```python
from build123d import *

# Parameters (mm, degrees)
EXTRUDE_1_DEPTH     = 2.5
SKETCH_2_W          = 15.8
SKETCH_2_H          = 6.5
EXTRUDE_2_DEPTH     = 1
FILLET_1_R          = 0.5
CUT_EXTRUDE_1_DEPTH = 12.419391402
SKETCH_4_W          = 21.55935693
SKETCH_4_H          = 12.890776674
SKETCH_4_W_2        = 6.1
SKETCH_4_H_2        = 6.5
CUT_EXTRUDE_2_DEPTH = 10
FILLET_2_R          = 0.5
CHAMFER_1_SIZE      = 0.5


with BuildPart() as part:
    # 草图1 → 凸台-拉伸1 (new body)
    with BuildSketch(Plane.XY):
        with BuildLine():
            Line((-9.05, -1.25), (-9.05, -3.45))
            ThreePointArc((-9.05, -3.45), (-8.713172798, -4.263172798), (-7.9, -4.6))
            Line((-7.9, -4.6), (7.9, -4.6))
            ThreePointArc((7.9, -4.6), (8.713172798, -4.263172798), (9.05, -3.45))
            Line((9.05, -3.45), (9.05, -1.25))
            ThreePointArc((9.05, -1.25), (8.713172798, -0.436827202), (7.9, -0.1))
            Line((7.9, -0.1), (-7.9, -0.1))
            ThreePointArc((-7.9, -0.1), (-8.713172798, -0.436827202), (-9.05, -1.25))
        make_face()
    extrude(amount=-EXTRUDE_1_DEPTH)

    # 草图2 → 凸台-拉伸2 (add)
    with BuildSketch(Plane(origin=(0, 0, -2.5), x_dir=(-1, 0, 0), z_dir=(0, 0, -1))):
        with Locations((0, -2.35)):
            Rectangle(SKETCH_2_W, SKETCH_2_H)
    extrude(amount=-EXTRUDE_2_DEPTH)

    # 圆角1
    fillet_1_edges = [part.edges().sort_by_distance(p)[0] for p in [
        (-7.9, 0.9, -2),
        (-7.9, -5.6, -2),
        (7.9, -5.6, -2),
        (7.9, 0.9, -2),
    ]]
    fillet(fillet_1_edges, radius=FILLET_1_R)

    # 草图3 → 切除-拉伸1 (cut, through all)
    with BuildSketch(Plane(origin=(0, 0.9, 0), x_dir=(1, 0, 0), z_dir=(0, 1, 0))):
        Polygon((8.475, 2.5), (9.05, 1.925), (9.05, 2.5), align=None)
        Polygon((-9.05, 1.925), (-9.05, 2.5), (-8.475, 2.5), align=None)
    extrude(amount=-CUT_EXTRUDE_1_DEPTH, mode=Mode.SUBTRACT)

    # 草图4 → 切除-拉伸2 (cut)
    with BuildSketch(Plane(origin=(0, 0, -2.5), x_dir=(-1, 0, 0), z_dir=(0, 0, -1))):
        with Locations((0, -2.35)):
            Rectangle(SKETCH_4_W, SKETCH_4_H)
        with Locations((0, -2.35)):
            Rectangle(SKETCH_4_W_2, SKETCH_4_H_2, mode=Mode.SUBTRACT)
    extrude(amount=-CUT_EXTRUDE_2_DEPTH, mode=Mode.SUBTRACT)

    # 圆角2
    fillet_2_edges = [part.edges().sort_by_distance(p)[0] for p in [
        (3.05, 0.9, -2),
        (-3.05, 0.9, -2),
        (3.05, -5.6, -2),
        (-3.05, -5.6, -2),
        (-3.05, -0.1, -0.75),
        (-3.05, -4.6, -0.75),
        (3.05, -0.1, -0.75),
        (3.05, -4.6, -0.75),
    ]]
    fillet(fillet_2_edges, radius=FILLET_2_R)

    # 倒角1
    chamfer_1_edges = [part.edges().sort_by_distance(p)[0] for p in [
        (0, -4.6, 0),
        (-3.05, -2.35, 0),
        (0, -0.1, 0),
        (3.05, -2.35, 0),
        (2.903553391, -0.246446609, 0),
        (-2.903553391, -0.246446609, 0),
        (2.903553391, -4.453553391, 0),
        (-2.903553391, -4.453553391, 0),
    ]]
    chamfer(chamfer_1_edges, length=CHAMFER_1_SIZE)


solid = part.part
```
CAD build for the part. Positions are in the model's coordinates, mm. A direction names the side the tool comes from. Give positions to 0.01 mm unless a question says otherwise; leave off trailing zeros. Order: outer loops, then holes, each group sorted by start corner. A loop starts at its lowest first (then second) coordinate and runs counter-clockwise, first axis right, second up.
(1) Saw through at B-B, the plane y = -3.75. Give the cut face in (x, z).
(2) Drill centre lines: L1, parallel to Y at x = -0.5, z = -1.2; L2, parallel to Z at x = -0.75, y = 0.5; L3, parallel to Z at x = 1, y = -0.5. Where is each one in solid material? Low to high.
(3) Saw through at D-D, the plane y = 0.25. Give the cut face in (x, z), then the cut area to 3 significant figures.
(4) Saw through at C-C, the plane z = -1.4. Give the cut face in (x, y).
(5) Saw through at A-A, the plane x = -0.5. Give the cut face in (y, z).
(6) Flat gauge pins, fed straight in: pin 1 (0.5 mm diameter, centred on x = 0.5, z = -1, fed in from -Y); pin 2 (1.6 mm diameter, centred on x = -1.5, y = -5, fed in from +Z); pin 3 (1 mm diameter, centred on x = 1, z = -0.5, fed in from +Y). Where does each tip first touch, or does it go through?
(7) Tool access for faces 1 (the flat face through (0, -0.1, -1)), 2 (the flat face through (0, -4.6, -1)), 3 (the flat face through (-3.05, -2, -2)): list every direction of +Z, -Z, +X, -X, +Y, -Y with a clear straight run to the whole face (end or side of a thin tool).
Results found:
1. outline: (-3.05, -2.5) - (3.05, -2.5) - (3.05, -0.5) - (2.55, 0) - (-2.55, 0) - (-3.05, -0.5) - close
2. L1: y = -4.6 to -0.1
2. L2: z = -2.5 to -1.5
2. L3: z = -2.5 to -0.1
3. outline: (-3.05, -2.5) - (3.05, -2.5) - (3.05, -1.5) - (-3.05, -1.5) - close
3. area: 6.10 mm2
4. outline: (-3.05, -4.1) arc R0.5 ccw to (-2.55, -4.6) - (2.55, -4.6) arc R0.5 ccw to (3.05, -4.1) - (3.05, -0.6) arc R0.5 ccw to (2.55, -0.1) - (-2.55, -0.1) arc R0.5 ccw to (-3.05, -0.6) - close
5. outline: (-5.6, -2.5) - (0.9, -2.5) - (0.9, -1.5) - (-0.1, -1.5) - (-0.1, -0.5) - (-0.6, 0) - (-4.1, 0) - (-4.6, -0.5) - (-4.6, -1.5) - (-5.6, -1.5) - close
6. pin 1: stops at y = -4.6
6. pin 2: stops at z = -0.1
6. pin 3: stops at y = -0.1
7. face 1: +Z, +X, -X, +Y
7. face 2: +Z, +X, -X, -Y
7. face 3: +Z, -Z, -X, +Y, -Y
